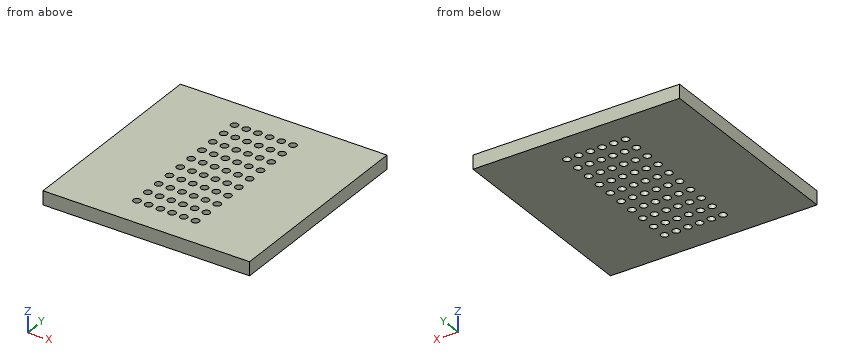
```python
from build123d import *

# Parameters (mm, degrees)
ESQUISSE1_W            = 30
ESQUISSE1_H            = 30
BASE_PLATE_DEPTH       = 2
SKETCH_PERFORATIONS_R  = 0.53
CUT_PERFORATIONS_DEPTH = 10


with BuildPart() as part:
    # Esquisse1 → Base_Plate (new body)
    with BuildSketch(Plane.XY):
        Rectangle(ESQUISSE1_W, ESQUISSE1_H)
    extrude(amount=BASE_PLATE_DEPTH)

    # Sketch_Perforations → Cut_Perforations (cut)
    with BuildSketch(Plane.XY.offset(2)):
        with Locations((-4.25, -10.64)):
            Circle(SKETCH_PERFORATIONS_R)
        with Locations((-4.25, -8.27)):
            Circle(SKETCH_PERFORATIONS_R)
        with Locations((-4.25, -5.91)):
            Circle(SKETCH_PERFORATIONS_R)
        with Locations((-4.25, -3.55)):
            Circle(SKETCH_PERFORATIONS_R)
        with Locations((-4.25, -1.18)):
            Circle(SKETCH_PERFORATIONS_R)
        with Locations((-4.25, 1.18)):
            Circle(SKETCH_PERFORATIONS_R)
        with Locations((-4.25, 3.55)):
            Circle(SKETCH_PERFORATIONS_R)
        with Locations((-4.25, 5.91)):
            Circle(SKETCH_PERFORATIONS_R)
        with Locations((-4.25, 8.27)):
            Circle(SKETCH_PERFORATIONS_R)
        with Locations((-4.25, 10.64)):
            Circle(SKETCH_PERFORATIONS_R)
        with Locations((-2.55, -10.64)):
            Circle(SKETCH_PERFORATIONS_R)
        with Locations((-2.55, -8.27)):
            Circle(SKETCH_PERFORATIONS_R)
        with Locations((-2.55, -5.91)):
            Circle(SKETCH_PERFORATIONS_R)
        with Locations((-2.55, -3.55)):
            Circle(SKETCH_PERFORATIONS_R)
        with Locations((-2.55, -1.18)):
            Circle(SKETCH_PERFORATIONS_R)
        with Locations((-2.55, 1.18)):
            Circle(SKETCH_PERFORATIONS_R)
        with Locations((-2.55, 3.55)):
            Circle(SKETCH_PERFORATIONS_R)
        with Locations((-2.55, 5.91)):
            Circle(SKETCH_PERFORATIONS_R)
        with Locations((-2.55, 8.27)):
            Circle(SKETCH_PERFORATIONS_R)
        with Locations((-2.55, 10.64)):
            Circle(SKETCH_PERFORATIONS_R)
        with Locations((-0.85, -10.64)):
            Circle(SKETCH_PERFORATIONS_R)
        with Locations((-0.85, -8.27)):
            Circle(SKETCH_PERFORATIONS_R)
        with Locations((-0.85, -5.91)):
            Circle(SKETCH_PERFORATIONS_R)
        with Locations((-0.85, -3.55)):
            Circle(SKETCH_PERFORATIONS_R)
        with Locations((-0.85, -1.18)):
            Circle(SKETCH_PERFORATIONS_R)
        with Locations((-0.85, 1.18)):
            Circle(SKETCH_PERFORATIONS_R)
        with Locations((-0.85, 3.55)):
            Circle(SKETCH_PERFORATIONS_R)
        with Locations((-0.85, 5.91)):
            Circle(SKETCH_PERFORATIONS_R)
        with Locations((-0.85, 8.27)):
            Circle(SKETCH_PERFORATIONS_R)
        with Locations((-0.85, 10.64)):
            Circle(SKETCH_PERFORATIONS_R)
        with Locations((0.85, -10.64)):
            Circle(SKETCH_PERFORATIONS_R)
        with Locations((0.85, -8.27)):
            Circle(SKETCH_PERFORATIONS_R)
        with Locations((0.85, -5.91)):
            Circle(SKETCH_PERFORATIONS_R)
        with Locations((0.85, -3.55)):
            Circle(SKETCH_PERFORATIONS_R)
        with Locations((0.85, -1.18)):
            Circle(SKETCH_PERFORATIONS_R)
        with Locations((0.85, 1.18)):
            Circle(SKETCH_PERFORATIONS_R)
        with Locations((0.85, 3.55)):
            Circle(SKETCH_PERFORATIONS_R)
        with Locations((0.85, 5.91)):
            Circle(SKETCH_PERFORATIONS_R)
        with Locations((0.85, 8.27)):
            Circle(SKETCH_PERFORATIONS_R)
        with Locations((0.85, 10.64)):
            Circle(SKETCH_PERFORATIONS_R)
        with Locations((2.55, -10.64)):
            Circle(SKETCH_PERFORATIONS_R)
        with Locations((2.55, -8.27)):
            Circle(SKETCH_PERFORATIONS_R)
        with Locations((2.55, -5.91)):
            Circle(SKETCH_PERFORATIONS_R)
        with Locations((2.55, -3.55)):
            Circle(SKETCH_PERFORATIONS_R)
        with Locations((2.55, -1.18)):
            Circle(SKETCH_PERFORATIONS_R)
        with Locations((2.55, 1.18)):
            Circle(SKETCH_PERFORATIONS_R)
        with Locations((2.55, 3.55)):
            Circle(SKETCH_PERFORATIONS_R)
        with Locations((2.55, 5.91)):
            Circle(SKETCH_PERFORATIONS_R)
        with Locations((2.55, 8.27)):
            Circle(SKETCH_PERFORATIONS_R)
        with Locations((2.55, 10.64)):
            Circle(SKETCH_PERFORATIONS_R)
        with Locations((4.25, -10.64)):
            Circle(SKETCH_PERFORATIONS_R)
        with Locations((4.25, -8.27)):
            Circle(SKETCH_PERFORATIONS_R)
        with Locations((4.25, -5.91)):
            Circle(SKETCH_PERFORATIONS_R)
        with Locations((4.25, -3.55)):
            Circle(SKETCH_PERFORATIONS_R)
        with Locations((4.25, -1.18)):
            Circle(SKETCH_PERFORATIONS_R)
        with Locations((4.25, 1.18)):
            Circle(SKETCH_PERFORATIONS_R)
        with Locations((4.25, 3.55)):
            Circle(SKETCH_PERFORATIONS_R)
        with Locations((4.25, 5.91)):
            Circle(SKETCH_PERFORATIONS_R)
        with Locations((4.25, 8.27)):
            Circle(SKETCH_PERFORATIONS_R)
        with Locations((4.25, 10.64)):
            Circle(SKETCH_PERFORATIONS_R)
    extrude(amount=-CUT_PERFORATIONS_DEPTH, mode=Mode.SUBTRACT)


solid = part.part
```
Model file for the job. Use its own axes, mm. Coordinates: 2 decimals unless noted, no trailing zeros. Loops run counter-clockwise (first coordinate to the right, second up) from the corner with the lowest first, then second, coordinate; pieces in that order, holes last. Notation, with made-up numbers: (4, 70.25) - (18, 70.25) arc R14 ccw to (18, 90.25) - close; hole circle Ø8 at (80, 56). An arc over 180 degrees is marked (long way). Answer as a JSON object with one key per item and string values. Group by question number.
(1) Cut at B-B (x = 0.85). State how many separate pieces and enclosed holes the cut face has, then the cut area to 3 significant figures.
(2) Cut at A-A (y = 1.18). Give the cut face in (x, z), then the cut area to 3 significant figures.
(3) Flat gauge pins, fed straight in: pin 1 (1.2 mm diameter, centred on x = -2.55, y = -5.91, fed in from +Z); pin 2 (1 mm diameter, centred on x = -4.25, y = -8.27, fed in from -Z). Where does each tip first touch, or does it go through?
Geometry says:
{
 "1": {"separate pieces": "11", "enclosed holes": "0", "area": "38.8 mm^2"},
 "2": {"outline": "(-15, 0) - (-4.78, 0) - (-4.78, 2) - (-15, 2) - close; (-3.72, 0) - (-3.08, 0) - (-3.08, 2) - (-3.72, 2) - close; (-2.02, 0) - (-1.38, 0) - (-1.38, 2) - (-2.02, 2) - close; (-0.32, 0) - (0.32, 0) - (0.32, 2) - (-0.32, 2) - close; (1.38, 0) - (2.02, 0) - (2.02, 2) - (1.38, 2) - close; (3.08, 0) - (3.72, 0) - (3.72, 2) - (3.08, 2) - close; (4.78, 0) - (15, 0) - (15, 2) - (4.78, 2) - close", "area": "47.3 mm^2"},
 "3": {"pin 1": "stops at z = 2", "pin 2": "passes through"}
}
